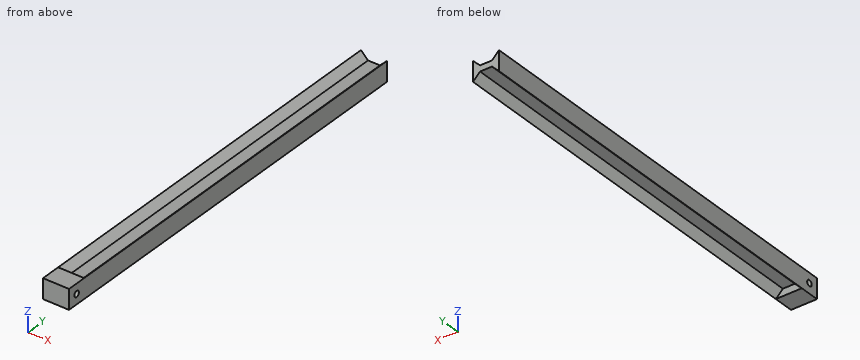
from build123d import *

# Parameters (mm, degrees)
BOSS_EXTRUDE1_DEPTH = 200
SKETCH2_W           = 13.071067812
SKETCH2_H           = 10
BOSS_EXTRUDE2_DEPTH = 10
SKETCH3_R           = 1.5
CUT_EXTRUDE1_DEPTH  = 30


with BuildPart() as part:
    # Sketch1 → Boss-Extrude1 (new body)
    with BuildSketch(Plane(origin=(0, 0, 0), x_dir=(1, 0, 0), z_dir=(0, 1, 0))):
        Polygon((0, 0), (-3.535533906, -3.535533906), (-9.535533906, -3.535533906), (-13.071067812, 0), (-13.071067812, -10), (-9.535533906, -6.464466094), (-3.535533906, -6.464466094), (0, -10), align=None)
    extrude(amount=BOSS_EXTRUDE1_DEPTH)

    # Sketch2 → Boss-Extrude2 (add)
    with BuildSketch(Plane.XZ):
        with Locations((-6.535533906, 5)):
            Rectangle(SKETCH2_W, SKETCH2_H)
    extrude(amount=BOSS_EXTRUDE2_DEPTH)

    # Sketch3 → Cut-Extrude1 (cut)
    with BuildSketch(Plane.ZY.offset(13.071067812)):
        with Locations((5, -5)):
            Circle(SKETCH3_R)
    extrude(amount=-CUT_EXTRUDE1_DEPTH, mode=Mode.SUBTRACT)


solid = part.part
Read the model definition and answer for the solid it produces. Units are mm, in the model's axes. Give positions to 0.01 mm unless a question says otherwise; leave off trailing zeros. Write each loop counter-clockwise with the first axis right and the second up, starting at its lowest first coordinate (ties: lowest second). Pieces come first, ordered by that corner, then holes. Notation, with made-up numbers: (-30, 57.25) - (-9, 57.25) arc R8 ccw to (-9, 61.25) - close; hole circle Ø3 at (-1, 29). An arc over 180 degrees is marked (long way). Answer in a Markdown table with one row per item. Add a question column.
Item 1: Section A-A, the plane y = 26 is taken. Write down the section's boundary in (x, z), and give its area (3 significant figures).
Item 2: Flat-ended cylindrical pins translate along their axes: P1, Ø1.8, axis at x = -5, z = 1, coming from the +Y side; P2, Ø1, axis at x = -8, y = 143, coming from the +Z side; P3, Ø5, axis at x = -7, y = 64, coming from the -Z side. Find the tip coordinate at first contact, or state that the pin passes through.
Item 3: Section B-B, the plane x = -6.5 is taken. Write down the section's boundary in (y, z), and give its area (3 significant figures).
Item 4: Find the intervals of material crossed by L1, parallel to Y at x = -3, z = 5; L2, parallel to Z at x = -4.5, y = 34.5; L3, parallel to Y at x = -5, z = 9.5, in increasing order.
Recorded:
| question | item | result |
|---|---|---|
| 1 | outline | (-13.07, 0) - (-9.54, 3.54) - (-3.54, 3.54) - (0, 0) - (0, 10) - (-3.54, 6.46) - (-9.54, 6.46) - (-13.07, 10) - close |
| 1 | area | 63.3 mm2 |
| 2 | P1 | stops at y = 0 |
| 2 | P2 | stops at z = 6.46 |
| 2 | P3 | stops at z = 3.54 |
| 3 | outline | (-10, 0) - (0, 0) - (0, 3.54) - (200, 3.54) - (200, 6.46) - (0, 6.46) - (0, 10) - (-10, 10) - close; hole circle Ø3 at (-5, 5) |
| 3 | area | 679 mm2 |
| 4 | L1 | y = -10 to -6.5, -3.5 to 200 |
| 4 | L2 | z = 3.54 to 6.46 |
| 4 | L3 | y = -10 to 0 |
